Geometry: final body of the model. Coordinates: model frame, mm. A direction names the side the tool comes from. Round coordinates to 2 decimals unless told otherwise and drop trailing zeros. Loops run counter-clockwise (first coordinate to the right, second up) from the corner with the lowest first, then second, coordinate; pieces in that order, holes last. Notation, with made-up numbers: (60.25, 49) - (81.25, 49) arc R18 cw to (81.25, 78) - close; hole circle Ø9 at (10, 54.5). An arc over 180 degrees is marked (long way). Return JSON: item names as keys, results as strings. Group by question number.
1. Section A-A on y = 0. Return loops of the section in (x, z), and give its area (3 significant figures).
2. Material intervals for probe 1 along X at (y, z) = (0, -0.5); probe 2 along Z at (x, y) = (14, 0.9), sorted ascending.
3. Section B-B on x = 0. Return loops of the section in (y, z).
4. Set-up query: faces 1 (the face through (1.29, 2.024, 0.993)), 2 (the face through (1.29, -2.024, -0.986)), 3 (the face through (0, -1, 2.5)). Return all of +Z, -Z, +X, -X, +Y, -Y with unobstructed straight access to the full face (end or side cutting, diameter ignored); none if empty.
5. Section D-D on x = -16.5. Return loops of the section in (y, z).
6. First-contact query: pin 1 Ø2 at (y, z) = (1.5, 0.5) entering from +X; pin 2 Ø3 at (x, y) = (22.5, -0.5) entering from +Z; pin 3 Ø1.5 at (y, z) = (1.5, -1) entering from +X; pin 4 Ø1.5 at (x, y) = (17.5, -0.5) entering from -Z. Flat tips, straight axial feed; report the tip coordinate or a pass-through.
7. Draft query along Y for faces 4 (the face through (-0.75, -0.03, 0.28)), 5 (the face through (16.2, -2.3, 0.2)), 6 (the face through (0, -1, -2)), 7 (the face through (16.63, 2.28, 0.25)). Return one class per face: +Y half, -Y half, draft (parallel to the pull), parting line (faces both ways), or undercut.
8. Section C-C on z = -1.3. Return loops of the section in (x, y), and give its area (3 significant figures).
from build123d import *

# Parameters (mm, degrees)
F0_R     = 0.75
F1_DEPTH = 0.5
F2_R     = 2.4
F2_R_2   = 0.75
F3_DEPTH = 2
F4_R     = 1
F5_R     = 2.4
F5_R_2   = 0.75
F6_DEPTH = 2


with BuildPart() as f1:
    # F0 (on Top) → F1 (new body)
    with BuildSketch(Plane.XY):
        with BuildLine():
            ThreePointArc((-32.0556782457, 1.0502037309), (-32.3727191455, 0.8866007898), (-32.5, 0.5533134684))
            Line((-32.5, 0.5533134684), (-32.5, -0.5533134684))
            ThreePointArc((-32.5, -0.5533134684), (-32.3727191455, -0.8866007898), (-32.0556782457, -1.0502037309))
            ThreePointArc((-32.0556782457, -1.0502037309), (-16.4153028407, -2.2906426773), (-0.7274094873, -2.5143248665))
            ThreePointArc((-0.7274094873, -2.5143248665), (0, -2.5077102626), (0.7274094873, -2.5143248665))
            ThreePointArc((0.7274094873, -2.5143248665), (16.4153028407, -2.2906426773), (32.0556782457, -1.0502037309))
            ThreePointArc((32.0556782457, -1.0502037309), (32.3727191455, -0.8866007898), (32.5, -0.5533134684))
            Line((32.5, -0.5533134684), (32.5, 0.5533134684))
            ThreePointArc((32.5, 0.5533134684), (32.3727191455, 0.8866007898), (32.0556782457, 1.0502037309))
            ThreePointArc((32.0556782457, 1.0502037309), (16.4153028407, 2.2906426773), (0.7274094872, 2.5143248666))
            ThreePointArc((0.7274094872, 2.5143248666), (0, 2.5077102626), (-0.7274094872, 2.5143248666))
            ThreePointArc((-0.7274094872, 2.5143248666), (-16.4153028407, 2.2906426773), (-32.0556782457, 1.0502037309))
        make_face()
        Circle(F0_R, mode=Mode.SUBTRACT)
    extrude(amount=F1_DEPTH)

    # F2 (on face) → F3 (join)
    with BuildSketch(Plane.XY.offset(0.5)):
        Circle(F2_R)
        Circle(F2_R_2, mode=Mode.SUBTRACT)
    extrude(amount=F3_DEPTH)

    # F4
    f4_edges = [f1.edges().sort_by_distance(p)[0] for p in [
        (-2.4, 0, 2.5),
    ]]
    fillet(f4_edges, radius=F4_R)

    # F5 (on face) → F6 (join)
    with BuildSketch(Plane(origin=(0, 0, 0), x_dir=(1, 0, 0), z_dir=(0, 0, -1))):
        Circle(F5_R)
        Circle(F5_R_2, mode=Mode.SUBTRACT)
    extrude(amount=F6_DEPTH)


solid = f1.part
Taken from the geometry:
{
 "1": {"outline": "(-32.5, 0) - (-2.4, 0) - (-2.4, -2) - (-0.75, -2) - (-0.75, 2.5) - (-1.4, 2.5) arc R1 ccw to (-2.4, 1.5) - (-2.4, 0.5) - (-32.5, 0.5) - close; (0.75, -2) - (2.4, -2) - (2.4, 0) - (32.5, 0) - (32.5, 0.5) - (2.4, 0.5) - (2.4, 1.5) arc R1 ccw to (1.4, 2.5) - (0.75, 2.5) - close", "area": "44.5 mm2"},
 "2": {"probe 1": "-2.4 to -0.75, 0.75 to 2.4", "probe 2": "0 to 0.5"},
 "3": {"outline": "(-2.51, 0) - (-2.4, 0) - (-2.4, -2) - (-0.75, -2) - (-0.75, 2.5) - (-1.4, 2.5) arc R1 ccw to (-2.4, 1.5) - (-2.4, 0.5) - (-2.51, 0.5) - close; (0.75, -2) - (2.4, -2) - (2.4, 0) - (2.51, 0) - (2.51, 0.5) - (2.4, 0.5) - (2.4, 1.5) arc R1 ccw to (1.4, 2.5) - (0.75, 2.5) - close"},
 "4": {"face 1": "+Z", "face 2": "-Z", "face 3": "+Z, +X, -X, +Y, -Y"},
 "5": {"outline": "(-2.29, 0) - (2.29, 0) - (2.29, 0.5) - (-2.29, 0.5) - close"},
 "6": {"pin 1": "x = 32.5", "pin 2": "z = 0.5", "pin 3": "x = 2.28", "pin 4": "z = 0"},
 "7": {"face 4": "undercut", "face 5": "-Y half", "face 6": "draft", "face 7": "+Y half"},
 "8": {"outline": "circle Ø4.8 at (0, 0); hole circle Ø1.5 at (0, 0)", "area": "16.3 mm2"}
}
